Print and shaded views of the part. All mm, measured from the part's lowest x, y and z. A direction names the side the tool comes from. Round coordinates to 2 decimals unless told otherwise and drop trailing zeros. Write each loop counter-clockwise with the first axis right and the second up, starting at its lowest first coordinate (ties: lowest second). Pieces come first, ordered by that corner, then holes. Notation, with made-up numbers: (-31.5, -39.5) -> (-10.5, -39.5) arc R26 ccw to (-10.5, -4.5) -> close; hole circle Ø8 at (60.5, 79). An arc over 180 degrees is marked (long way). Return JSON: item names as keys, results as strings. Group by question number.
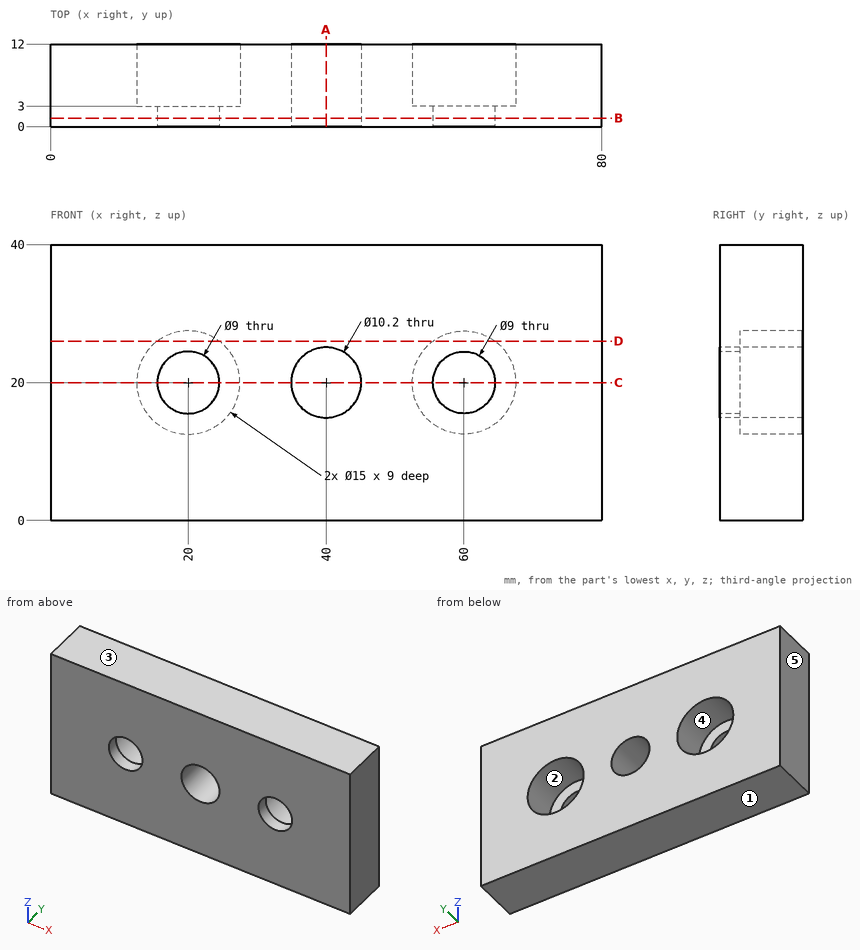
Item 1: Cut at A-A (x = 40). Write the cut outline in (y, z), then the cut area to 3 significant figures.
Item 2: Flat gauge pins, fed straight in: P1, Ø5.5, axis at x = 20, z = 20, coming from the -Y side; P2, Ø4.5, axis at x = 59.5, z = 23.5, coming from the +Y side. Where does each tip first touch, or does it go through?
Item 3: Wall check: L1, parallel to X at y = 1.6, z = 20; L2, parallel to X at y = 9.5, z = 20; L3, parallel to X at y = 4.75, z = 25.5. Give the ranges that are in metal, low to high.
Item 4: Two-plate mould, pull along X, no slides. Class the marked faces 3, 4 and 5: released by +X, released by -X, zero draft, split by the parting line, or undercut.
Item 5: Cut at C-C (z = 20). Write the cut outline in (x, y).
Item 6: Which spindle directions (+Z, -Z, +X, -X, +Y, -Y) get a long thin tool onto all of the face, cutting with end or side? Do the marked faces 1 and 2. Say none if no direction does.
Item 7: Cut at D-D (z = 26). Write the cut outline in (x, y), then the cut area to 3 significant figures.
Item 8: Cut at B-B (y = 1.25). Write the cut outline in (x, z), then the cut area to 3 significant figures.
Checks:
{
 "1": {"outline": "(0, 0) -> (12, 0) -> (12, 14.9) -> (0, 14.9) -> close; (0, 25.1) -> (12, 25.1) -> (12, 40) -> (0, 40) -> close", "area": "358 mm2"},
 "2": {"P1": "passes through", "P2": "stops at y = 3"},
 "3": {"L1": "x = 0 to 15.5, 24.5 to 34.9, 45.1 to 55.5, 64.5 to 80", "L2": "x = 0 to 12.5, 27.5 to 34.9, 45.1 to 52.5, 67.5 to 80", "L3": "x = 0 to 14.9, 25.1 to 54.9, 65.1 to 80"},
 "4": {"face 3": "zero draft", "face 4": "undercut", "face 5": "released by -X"},
 "5": {"outline": "(0, 0) -> (15.5, 0) -> (15.5, 3) -> (12.5, 3) -> (12.5, 12) -> (0, 12) -> close; (24.5, 0) -> (34.9, 0) -> (34.9, 12) -> (27.5, 12) -> (27.5, 3) -> (24.5, 3) -> close; (45.1, 0) -> (55.5, 0) -> (55.5, 3) -> (52.5, 3) -> (52.5, 12) -> (45.1, 12) -> close; (64.5, 0) -> (80, 0) -> (80, 12) -> (67.5, 12) -> (67.5, 3) -> (64.5, 3) -> close"},
 "6": {"face 1": "-Z, +X, -X, +Y, -Y", "face 2": "+Y"},
 "7": {"outline": "(0, 0) -> (80, 0) -> (80, 12) -> (64.5, 12) -> (64.5, 3) -> (55.5, 3) -> (55.5, 12) -> (24.5, 12) -> (24.5, 3) -> (15.5, 3) -> (15.5, 12) -> (0, 12) -> close", "area": "798 mm2"},
 "8": {"outline": "(0, 0) -> (80, 0) -> (80, 40) -> (0, 40) -> close; hole circle Ø9 at (20, 20); hole circle Ø10.2 at (40, 20); hole circle Ø9 at (60, 20)", "area": "2,990 mm2"}
}
